```python
from build123d import *

# Parameters (mm, degrees)
SZKIC2_R                    = 10
DODANIE_WYCI_GNI_CIE2_DEPTH = 20


with BuildPart() as part:
    # Szkic2 → Dodanie-wyciągnięcie2 (new body)
    with BuildSketch(Plane.XY):
        with BuildLine():
            Line((0, 185.8153975), (0, 200))
            Line((0, 200), (300, 200))
            Line((300, 200), (300, 179.99999))
            Line((300, 179.99999), (268.100984266, 179.99999))
            Line((268.100984266, 179.99999), (150.537685313, 112.968737031))
            Line((150.537685313, 112.968737031), (55.152827757, 17.668229265))
            ThreePointArc((55.152827757, 17.668229265), (30.970417819, 9.307465427), (9.446642737, 23.142870322))
            ThreePointArc((9.446642737, 23.142870322), (8.323346954, 39.404883236), (20.969056487, 49.690839091))
            ThreePointArc((20.969056487, 49.690839091), (30.26105361, 50.929938535), (39.634727212, 50.825913662))
            ThreePointArc((39.634727212, 50.825913662), (49.37359719, 51.953421869), (57.922039747, 56.753525311))
            Line((57.922039747, 56.753525311), (114.485527726, 113.266993629))
            ThreePointArc((114.485527726, 113.266993629), (122.461819258, 123.951300931), (127.060971476, 136.466229937))
            Line((127.060971476, 136.466229937), (132.025285125, 156.762570766))
            ThreePointArc((132.025285125, 156.762570766), (130.65411111, 167.466839441), (122.461819258, 174.491641238))
            Line((122.461819258, 174.491641238), (83.453647812, 177.186358886))
            ThreePointArc((83.453647812, 177.186358886), (75.274757646, 176.24414951), (67.979862212, 172.427540613))
            ThreePointArc((67.979862212, 172.427540613), (61.096304048, 166.616485937), (54.641338034, 160.332765448))
            ThreePointArc((54.641338034, 160.332765448), (48.563505303, 154.928947374), (41.697006274, 150.570909792))
            ThreePointArc((41.697006274, 150.570909792), (20.320793886, 150.001184012), (6.859784063, 166.616485937))
            Line((6.859784063, 166.616485937), (6.859784063, 181.256700403))
            ThreePointArc((6.859784063, 181.256700403), (5.949401229, 184.069477829), (3.56355164, 185.8153975))
            Line((3.56355164, 185.8153975), (0, 185.8153975))
        make_face()
        with Locations((30.431430438, 29.443458524)):
            Circle(SZKIC2_R, mode=Mode.SUBTRACT)
        with Locations((30.431430438, 169.443458524)):
            Circle(SZKIC2_R, mode=Mode.SUBTRACT)
    extrude(amount=DODANIE_WYCI_GNI_CIE2_DEPTH)


solid = part.part
```
For this review, take the finished solid that the model builds, in its own axes (mm). A direction names the side the tool comes from. Round coordinates to 2 decimals unless told otherwise and drop trailing zeros. Loops run counter-clockwise (first coordinate to the right, second up) from the corner with the lowest first, then second, coordinate; pieces in that order, holes last.
(1) We need section B-B (x = 111.5). Give the boundary of the cut face in (y, z), plus the area to 3 significant figures.
Returned:
outline: (73.97, 0) - (110.28, 0) - (110.28, 20) - (73.97, 20) - close; (175.25, 0) - (200, 0) - (200, 20) - (175.25, 20) - close
area: 1,220 mm2
(2) Tool access review of faces 1 (the cylindrical face through (61.19, 166.7, 9.86)), 2 (the flat face through (6.86, 174, 10)), 3 (the cylindrical face through (122.372, 123.787, 9.86)): name each direction out of +Z, -Z, +X, -X, +Y, -Y from which nothing blocks a thin tool from reaching the whole face with its end or side.
Returned:
face 1: +Z, -Z
face 2: +Z, -Z, -X, -Y
face 3: +Z, -Z, -X
(3) Mouldability with a two-part tool opening along Y and no side actions: class faces 4 (the cylindrical face through (75.39, 176.28, 9.86)), 5 (the flat face through (103.23, 175.82, 9.86)), 6 (the flat face through (300, 190, 10)), 7 (the flat face through (284, 180, 10)) as released by +Y, released by -Y, zero draft, split by the parting line, or undercut.
Returned:
face 4: undercut
face 5: undercut
face 6: zero draft
face 7: released by -Y
(4) Clearance check with flat-ended pins moving along their axes: P1, Ø12, axis at y = 155.5, z = 4.5, coming from the +X side; P2, Ø3, axis at y = 156.5, z = 11, coming from the -X side; P3, Ø10, axis at y = 126, z = 8.5, coming from the -X side; P4, Ø3, axis at x = 132, y = 156.5, coming from the -Z side. State where each tip first meets the part, or that it passes through.
Returned:
P1: stops at x = 235.65
P2: stops at x = 10.7
P3: stops at x = 120.72
P4: stops at z = 0
(5) We need section C-C (z = 13.5). Give the boundary of the cut face in (x, y).
Returned:
outline: (0, 185.82) - (3.56, 185.82) arc R4.8 cw to (6.86, 181.26) - (6.86, 166.62) arc R24.17 ccw to (41.7, 150.57) arc R50.5 ccw to (54.64, 160.33) arc R127.19 cw to (67.98, 172.43) arc R22.54 cw to (83.45, 177.19) - (122.46, 174.49) arc R15.03 cw to (132.03, 156.76) - (127.06, 136.47) arc R46.28 cw to (114.49, 113.27) - (57.92, 56.75) arc R24.9 cw to (39.63, 50.83) arc R65.31 ccw to (20.97, 49.69) arc R17.7 ccw to (9.45, 23.14) arc R29.29 ccw to (55.15, 17.67) - (150.54, 112.97) - (268.1, 180) - (300, 180) - (300, 200) - (0, 200) - close; hole circle Ø20 at (30.43, 29.44); hole circle Ø20 at (30.43, 169.44)
(6) We need section A-A (y = 35). Give the boundary of the cut face in (x, z), plus the area to 3 significant figures.
Returned:
outline: (7.06, 0) - (22.12, 0) - (22.12, 20) - (7.06, 20) - close; (38.75, 0) - (72.5, 0) - (72.5, 20) - (38.75, 20) - close
area: 976 mm2
(7) Wall thickness on line 1 along Y through (x, z) = (30.5, 16.25); line 2 along Y through (x, z) = (74.5, 6.5); line 3 along X through (y, z) = (150.5, 12.75): over which ranges is each line inside the solid? List them lowest first.
Returned:
line 1: y = 9.37 to 19.44, 39.44 to 50.94, 147.78 to 159.44, 179.44 to 200
line 2: y = 37 to 73.32, 175.99 to 200
line 3: x = 19.3 to 41.56, 130.49 to 216.36
(8) We need section D-D (x = 276.5). Give the boundary of the cut face in (y, z), plus the area to 3 significant figures.
Returned:
outline: (180, 0) - (200, 0) - (200, 20) - (180, 20) - close
area: 400 mm2
